Can you work these out from the drawing? Everything is in mm from the part's minimum corner. A direction names the side the tool comes from. Give positions to 0.01 mm unless a question says otherwise; leave off trailing zeros. Write each loop counter-clockwise with the first axis right and the second up, starting at its lowest first coordinate (ties: lowest second). Pieces come first, ordered by that corner, then holes. Notation, with made-up numbers: (-26, 73.5) -> (-7, 73.5) arc R13 ccw to (-7, 86.5) -> close; hole circle Ø2 at (55, 37). An arc over 180 degrees is marked (long way). Return JSON: item names as keys, results as strings.
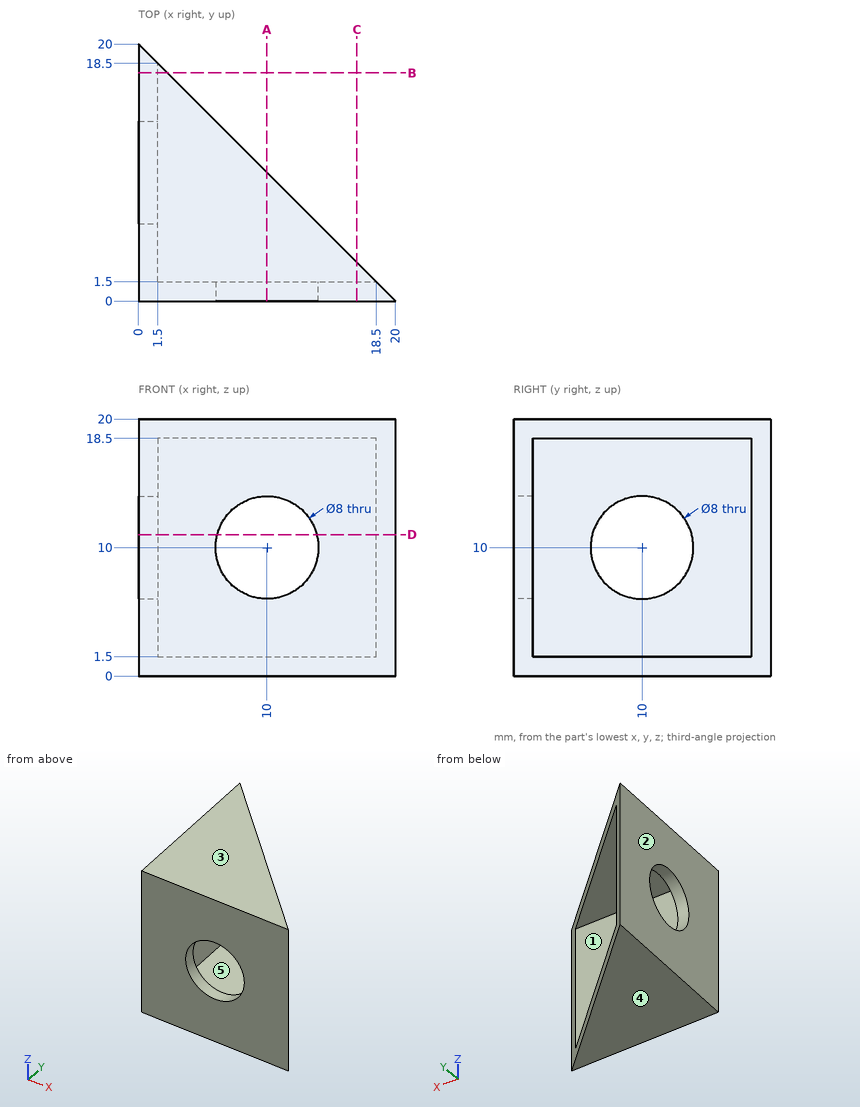
1. Suppose I cut it at C-C, the plane x = 17. List the corners of the cut face in (y, z) for me.
Taken from the geometry:
{"outline": "(0, 0) -> (3, 0) -> (3, 1.5) -> (1.5, 1.5) -> (1.5, 18.5) -> (3, 18.5) -> (3, 20) -> (0, 20) -> close"}
2. If we mould it in two halves opening along Z, with no side actions, what happens to the marked faces 1, 2 and 3? For each: released by +Z, released by -Z, zero draft, split by the parting line, or undercut.
Taken from the geometry:
{"face 1": "undercut", "face 2": "zero draft", "face 3": "released by +Z"}
3. Suppose I cut it at A-A, the plane x = 10. List the corners of the cut face in (y, z) for me, and give its area (3 significant figures).
Taken from the geometry:
{"outline": "(0, 0) -> (10, 0) -> (10, 1.5) -> (1.5, 1.5) -> (1.5, 6) -> (0, 6) -> close; (0, 14) -> (1.5, 14) -> (1.5, 18.5) -> (10, 18.5) -> (10, 20) -> (0, 20) -> close", "area": "43.5 mm²"}
4. If I drill on line 1 (Z direction, x = 7, y = 7); line 2 (X direction, y = 15.5, z = 4.5); line 3 (Z direction, x = 10, y = 0.55), over which ranges is the centre line in solid material (lowest first)? Write a range as [from, to].
Taken from the geometry:
{"line 1": "z = [0, 1.5], [18.5, 20]", "line 2": "x = [0, 1.5]", "line 3": "z = [0, 6], [14, 20]"}
5. For pin 1 Ø5 at (y, z) = (6.5, 13) entering from +X; pin 2 Ø5 at (x, y) = (13, 9.5) entering from -Z; pin 3 Ø1.5 at (x, z) = (15, 4) entering from +Y; pin 4 Ø5 at (y, z) = (10, 10) entering from -X, each with a flat end and sliding along its axis, tell me the tip position at first contact or that it passes through.
Taken from the geometry:
{"pin 1": "stops at x = 1.5", "pin 2": "stops at z = 0", "pin 3": "stops at y = 1.5", "pin 4": "passes through"}
6. Suppose I cut it at D-D, the plane z = 11. List the corners of the cut face in (x, y) for me.
Taken from the geometry:
{"outline": "(0, 0) -> (6.13, 0) -> (6.13, 1.5) -> (1.5, 1.5) -> (1.5, 6.13) -> (0, 6.13) -> close; (0, 13.87) -> (1.5, 13.87) -> (1.5, 18.5) -> (0, 20) -> close; (13.87, 0) -> (20, 0) -> (18.5, 1.5) -> (13.87, 1.5) -> close"}
7. Suppose I cut it at B-B, the plane y = 17.75. List the corners of the cut face in (x, z) for me, and give its area (4 significant figures).
Taken from the geometry:
{"outline": "(0, 0) -> (2.25, 0) -> (2.25, 1.5) -> (1.5, 1.5) -> (1.5, 18.5) -> (2.25, 18.5) -> (2.25, 20) -> (0, 20) -> close", "area": "32.25 mm²"}
8. Which directions (+Z, -Z, +X, -X, +Y, -Y) give clear straight access to the entire face, cutting with the end or side of a thin tool? Please do the marked faces 4 and 5.
Taken from the geometry:
{"face 4": "-Z, +X, -X, +Y, -Y", "face 5": "+X, +Y"}
